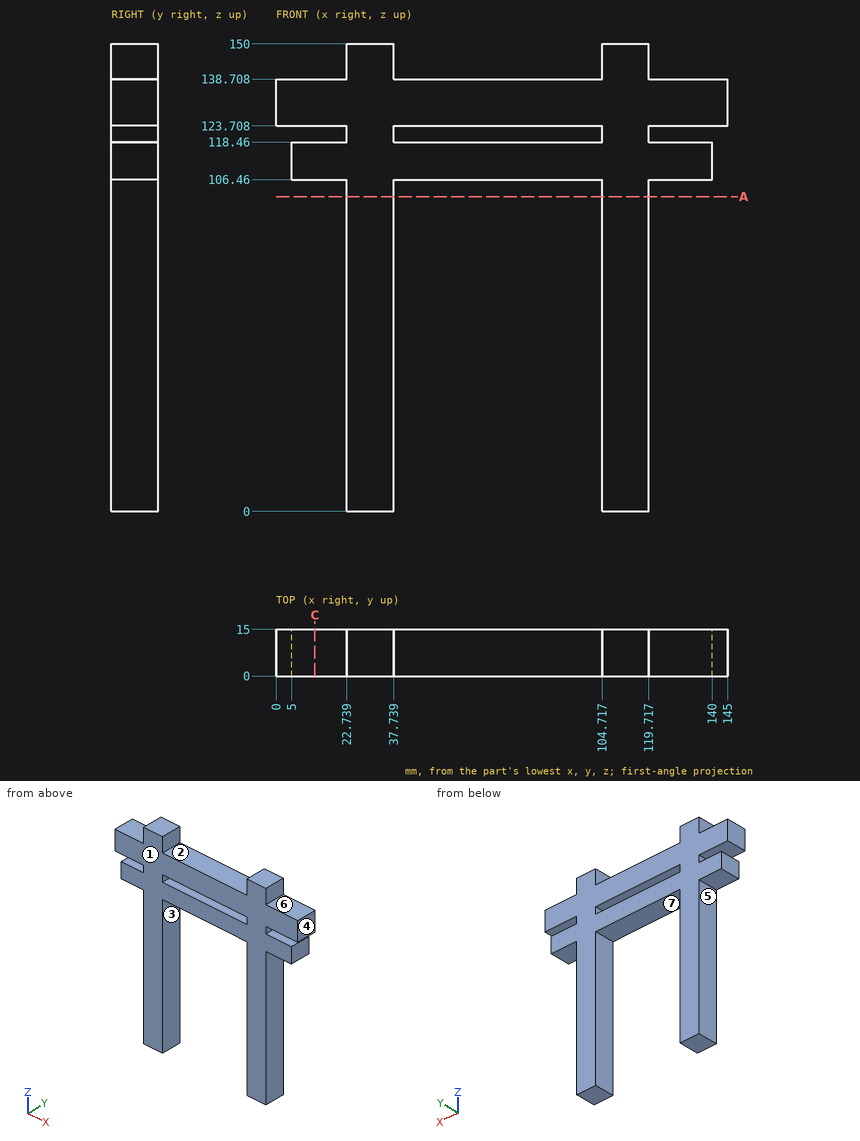
Verification items for this drawing (mm, ordinates from the low corner). A direction names the side the tool comes from. Give positions to 0.01 mm unless a question says otherwise; leave off trailing zeros. Write each loop counter-clockwise with the first axis right and the second up, starting at its lowest first coordinate (ties: lowest second). Pieces come first, ordered by that corner, then holes.
1) Access from +Z, -Z, +X, -X, +Y, -Y to the whole of each face (thin tool, end or side, straight path). Record for the marked faces 5, 6 and 7.
2) Gauge pin test, flat ends, axial feed: pin 1 (4.5 mm diameter, centred on x = 15.5, y = 6, fed in from -Z); pin 2 (5 mm diameter, centred on y = 11.5, z = 16.5, fed in from +X); pin 3 (7.5 mm diameter, centred on x = 79, y = 4, fed in from +Z); pin 4 (1 mm diameter, centred on x = 38.5, z = 47, fed in from -Y). Record the tip position at first contact, or that the pin passes through.
3) Section check A-A, the plane z = 101. Record the boundary of the cut face in (x, y), and give its area (3 significant figures).
4) Material ranges on L1, parallel to Z at x = 20, y = 10.75; L2, parallel to X at y = 1.5, z = 7.5; L3, parallel to X at y = 7, z = 107, recorded low to high.
5) Section check C-C, the plane x = 12.5. Record the boundary of the cut face in (y, z), and give its area (3 significant figures).
6) Release check for a two-part mould opening along X. For the marked faces 1, 2, 3 and 4 record: pulls with the +X half, pulls with the -X half, needs draft (parallel to the pull), parting line crosses it, or undercut.
Computed:
1. face 5: -Z, -X, +Y, -Y
1. face 6: +Z, +X, +Y, -Y
1. face 7: -Z, +Y, -Y
2. pin 1: stops at z = 106.46
2. pin 2: stops at x = 119.72
2. pin 3: stops at z = 138.71
2. pin 4: passes through
3. outline: (22.74, 0) - (37.74, 0) - (37.74, 15) - (22.74, 15) - close; (104.72, 0) - (119.72, 0) - (119.72, 15) - (104.72, 15) - close
3. area: 450 mm2
4. L1: z = 106.46 to 118.46, 123.71 to 138.71
4. L2: x = 22.74 to 37.74, 104.72 to 119.72
4. L3: x = 5 to 140
5. outline: (0, 106.46) - (15, 106.46) - (15, 118.46) - (0, 118.46) - close; (0, 123.71) - (15, 123.71) - (15, 138.71) - (0, 138.71) - close
5. area: 405 mm2
6. face 1: needs draft
6. face 2: undercut
6. face 3: undercut
6. face 4: pulls with the +X half
